Solid Edge part; units mm, degrees
sketch "Sketch1" plane through (0, 0, 0) normal (0, 0, 1) x (1, 0, 0)
  line L0 (-6.1009, 4.0673) -> (-6.5728, -3.2499)
  line L1 (-6.5728, -3.2499) -> (-0.4719, -7.3171)
  line L2 (-0.4719, -7.3171) -> (6.1009, -4.0673)
  line L3 (6.1009, -4.0673) -> (6.5728, 3.2499)
  line L4 (6.5728, 3.2499) -> (0.4719, 7.3171)
  line L5 (0.4719, 7.3171) -> (-6.1009, 4.0673)
extrude "Protrusion1" add sketch "Sketch1" against normal blind 104
sketch "Sketch2" plane through (0, 0, -2) normal (0, 0, 1) x (-0.8964, -0.4432, 0)
  circle A0 centre (0, 0) radius 5.5
  circle A1 centre (0, 0) radius 13.1424
extrude "ExtrudedCutout_1" cut sketch "Sketch2" against normal blind 2
sketch "Sketch3" plane through (0, 0, -102) normal (0, 0, -1) x (0.8964, 0.4432, 0)
  circle A0 centre (0, 0) radius 5.5
  circle A1 centre (0, 0) radius 13.1424
extrude "ExtrudedCutout_2" cut sketch "Sketch3" against normal blind 2
properties part number "BumbleB0660"
CAD build for the part. Positions are in the model's coordinates, mm. A direction names the side the tool comes from. Round coordinates to 2 decimals unless told otherwise and drop trailing zeros. Write each loop counter-clockwise with the first axis right and the second up, starting at its lowest first coordinate (ties: lowest second). Pieces come first, ordered by that corner, then holes.
(1) Slice it at B-B, the plane z = -98. Write the cut outline in (x, y), and give its area (3 significant figures).
(2) Slice it at C-C, the plane y = 0. Write the cut outline in (x, z), and give its area (3 significant figures).
(3) Probe line 1 along Z through (x, y) = (-6, 2.5); line 2 along X through (y, z) = (-6, -37); line 3 along X through (y, z) = (-4.5, -80). List the from-to ranges inside material, lowest first.
(4) Drop flat-ended pins along their axis: P1, Ø1, axis at x = 0, y = -5.5, coming from the +Z side; P2, Ø1, axis at y = 4, z = -14.5, coming from the +X side; P3, Ø2, axis at x = -4, z = -67.5, coming from the -Y side. Give the stop position or say it passes through.
(5) 3-axis set-ups, long thin cutter, end or side, ignore diameter. For faces 1 (the face through (-5, -3, -4)), 2 (the face through (-2.8, 5.7, -103)): which of +Z, -Z, +X, -X, +Y, -Y reach the whole face in a straight line?
(6) Slice it at A-A, the plane x = -3. Write the cut outline in (y, z), and give its area (3 significant figures).
From the geometry:
1. outline: (-6.57, -3.25) - (-0.47, -7.32) - (6.1, -4.07) - (6.57, 3.25) - (0.47, 7.32) - (-6.1, 4.07) - close
1. area: 140 mm2
2. outline: (-6.36, -104) - (6.36, -104) - (6.36, -102) - (5.5, -102) - (5.5, -100) - (6.36, -100) - (6.36, -4) - (5.5, -4) - (5.5, -2) - (6.36, -2) - (6.36, 0) - (-6.36, 0) - (-6.36, -2) - (-5.5, -2) - (-5.5, -4) - (-6.36, -4) - (-6.36, -100) - (-5.5, -100) - (-5.5, -102) - (-6.36, -102) - close
2. area: 1,320 mm2
3. line 1: z = -104 to -102, -100 to -4, -2 to 0
3. line 2: x = -2.45 to 2.19
3. line 3: x = -4.7 to 5.23
4. P1: stops at z = 0
4. P2: stops at x = 6.2
4. P3: stops at y = -5.63
5. face 1: none
5. face 2: +Z, -Z, -X, +Y
6. outline: (-5.63, -104) - (5.6, -104) - (5.6, -102) - (4.61, -102) - (4.61, -100) - (5.6, -100) - (5.6, -4) - (4.61, -4) - (4.61, -2) - (5.6, -2) - (5.6, 0) - (-5.63, 0) - (-5.63, -2) - (-4.61, -2) - (-4.61, -4) - (-5.63, -4) - (-5.63, -100) - (-4.61, -100) - (-4.61, -102) - (-5.63, -102) - close
6. area: 1,160 mm2
